Geometry: see drawing. Coordinates: mm, zero at the bounding-box minimum. A direction names the side the tool comes from. Round coordinates to 2 decimals unless told otherwise and drop trailing zeros. Loops run counter-clockwise (first coordinate to the right, second up) from the corner with the lowest first, then second, coordinate; pieces in that order, holes last.
(1) Cut plane B-B, the plane x = 1.5. Output: boundary loops of the cut face in (y, z) (1 decimal).
(2) Line query: line 1 (Z direction, x = 8.25, y = 16); line 2 (X direction, y = 2, z = 22); line 3 (Z direction, x = 2, y = 9). Output: solid intervals per line, ascending.
(3) Access query for the marked faces 1 and 2. Directions: +Z, -Z, +X, -X, +Y, -Y. A direction counts if a zero-diameter tool reaches every point of the face in a straight line with its end or side. Return the directions, or none.
(4) Draft query along Z for the marked faces 3, 4 and 5. Return one class per face: released by +Z, released by -Z, zero draft, split by the parting line, or undercut.
(5) Cut plane C-C, the plane x = 8.25. Output: boundary loops of the cut face in (y, z), and give its area (3 significant figures).
(6) Cut plane A-A, the plane y = 10.16. Output: boundary loops of the cut face in (x, z) (1 decimal).
(7) Cut plane D-D, the plane y = 22.86. Output: boundary loops of the cut face in (x, z) (1 decimal).
(8) First-contact query: pin 1 Ø6 at (y, z) = (11, 23.5) entering from +X. Flat tip, straight axial feed; report the tip coordinate or a pass-through.
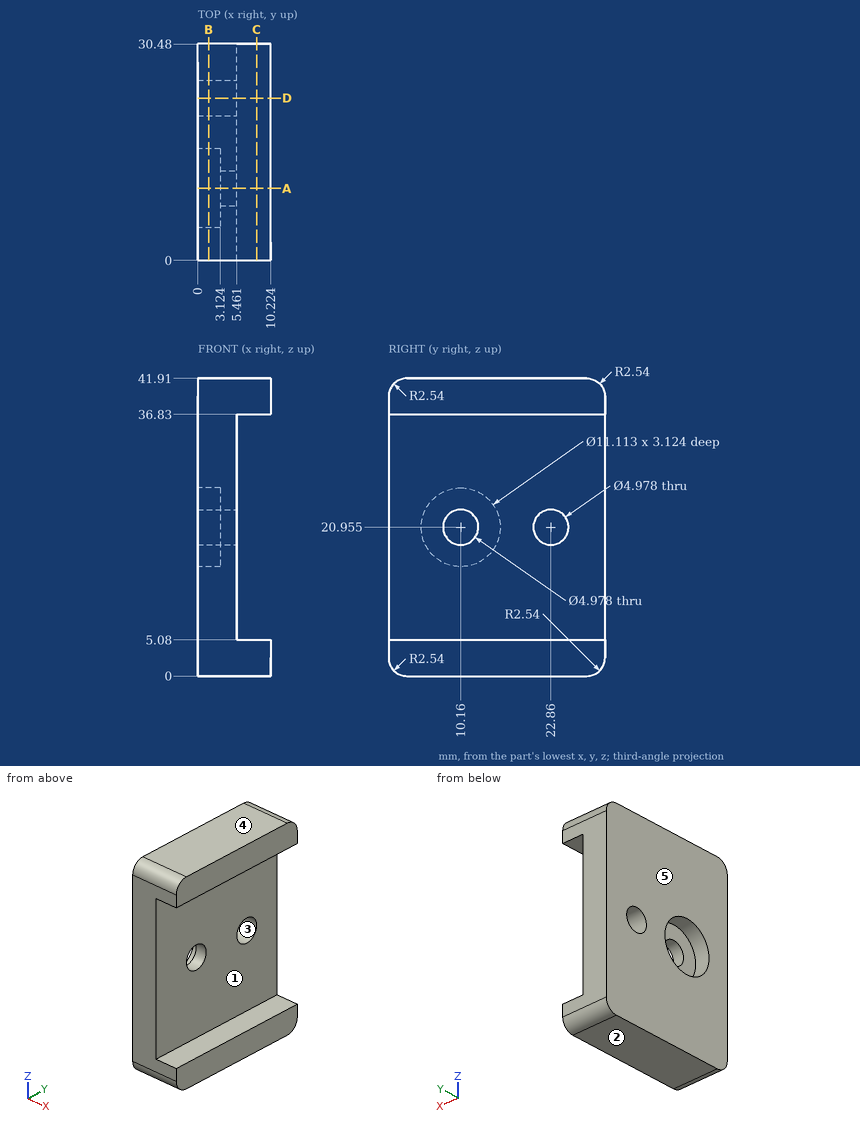
Reported:
1. outline: (0, 2.5) arc R2.5 ccw to (2.5, 0) - (27.9, 0) arc R2.5 ccw to (30.5, 2.5) - (30.5, 39.4) arc R2.5 ccw to (27.9, 41.9) - (2.5, 41.9) arc R2.5 ccw to (0, 39.4) - close; hole circle Ø11.1 at (10.2, 21); hole circle Ø5 at (22.9, 21)
2. line 1: z = 0 to 5.08, 36.83 to 41.91
2. line 2: x = 0 to 5.46
2. line 3: z = 0 to 15.52, 26.39 to 41.91
3. face 1: +X, +Y, -Y
3. face 2: -Z, +X, -X, +Y, -Y
4. face 3: undercut
4. face 4: released by +Z
4. face 5: zero draft
5. outline: (0, 2.54) arc R2.54 ccw to (2.54, 0) - (27.94, 0) arc R2.54 ccw to (30.48, 2.54) - (30.48, 5.08) - (0, 5.08) - close; (0, 36.83) - (30.48, 36.83) - (30.48, 39.37) arc R2.54 ccw to (27.94, 41.91) - (2.54, 41.91) arc R2.54 ccw to (0, 39.37) - close
5. area: 304 mm2
6. outline: (0, 0) - (10.2, 0) - (10.2, 5.1) - (5.5, 5.1) - (5.5, 18.5) - (3.1, 18.5) - (3.1, 15.4) - (0, 15.4) - close; (0, 26.5) - (3.1, 26.5) - (3.1, 23.4) - (5.5, 23.4) - (5.5, 36.8) - (10.2, 36.8) - (10.2, 41.9) - (0, 41.9) - close
7. outline: (0, 0) - (10.2, 0) - (10.2, 5.1) - (5.5, 5.1) - (5.5, 18.5) - (0, 18.5) - close; (0, 23.4) - (5.5, 23.4) - (5.5, 36.8) - (10.2, 36.8) - (10.2, 41.9) - (0, 41.9) - close
8. pin 1: stops at x = 5.46
